from build123d import *

# Parameters (mm, degrees)
SKETCH_1_W                   = 80
SKETCH_1_H                   = 105
SKETCH_1_R                   = 4.5
EXTRUDE_1_DEPTH              = 15
HOLE_WIZARD_M8_1_D           = 6.8
HOLE_WIZARD_M8_1_DEPTH       = 22.25
HOLE_WIZARD_M8_1_CSINK_D     = 8.05
HOLE_WIZARD_M8_1_CSINK_ANGLE = 90
HOLE_WIZARD_M8_1_TIP         = 2.042926105


with BuildPart() as part:
    # 草图1 → 凸台-拉伸1 (new body)
    with BuildSketch(Plane.XY):
        Rectangle(SKETCH_1_W, SKETCH_1_H)
        with Locations((-30, -12.5)):
            Circle(SKETCH_1_R, mode=Mode.SUBTRACT)
        with Locations((30, -12.5)):
            Circle(SKETCH_1_R, mode=Mode.SUBTRACT)
        with Locations((30, -42.5)):
            Circle(SKETCH_1_R, mode=Mode.SUBTRACT)
        with Locations((-30, -42.5)):
            Circle(SKETCH_1_R, mode=Mode.SUBTRACT)
    extrude(amount=EXTRUDE_1_DEPTH)

    # M8 螺纹孔1
    with Locations(Plane(origin=(-32, 52.5, 7.5), x_dir=(0, 0, 1), z_dir=(0, 1, 0))):
        with Locations((0, 0), (0, 64)):
            CounterSinkHole(HOLE_WIZARD_M8_1_D / 2, HOLE_WIZARD_M8_1_CSINK_D / 2, depth=HOLE_WIZARD_M8_1_DEPTH, counter_sink_angle=HOLE_WIZARD_M8_1_CSINK_ANGLE)
            with Locations((0, 0, -(HOLE_WIZARD_M8_1_DEPTH + HOLE_WIZARD_M8_1_TIP / 2))):  # 118° drill point
                Cone(0, HOLE_WIZARD_M8_1_D / 2, HOLE_WIZARD_M8_1_TIP, mode=Mode.SUBTRACT)


solid = part.part
Read the model definition and answer for the solid it produces. Units are mm, in the model's axes. A direction names the side the tool comes from. Round coordinates to 2 decimals unless told otherwise and drop trailing zeros. Order: outer loops, then holes, each group sorted by start corner. A loop starts at its lowest first (then second) coordinate and runs counter-clockwise, first axis right, second up.
1) Flat-ended cylindrical pins translate along their axes: pin 1 (8 mm diameter, centred on x = -30, y = -42.5, fed in from -Z); pin 2 (8 mm diameter, centred on x = 32, z = 7.5, fed in from +Y) (3 decimals); pin 3 (14.5 mm diameter, centred on x = 30, y = -42.5, fed in from -Z); pin 4 (1 mm diameter, centred on x = 30.5, z = 8.5, fed in from +Y). Find the tip coordinate at first contact, or state that the pin passes through.
2) The part is cut by section D-D on x = -30. Give the number of separate pieces and of enclosed holes in the cut face, plus the area to 3 significant figures.
3) The mould has two halves that part along Y. Classify faces 1 (the face through (-1, 1, 0)), 2 (the face through (-1, 52.5, 7)), 3 (the face through (-27.92, -46.49, 7.4)): released by +Y, released by -Y, zero draft, split by the parting line, or undercut.
4) The part is cut by section A-A on y = 37.5. Write down the section's boundary in (x, z).
5) The part is cut by section C-C on y = -42.5. Write down the section's boundary in (x, z).
6) The part is cut by section B-B on z = 13. Write down the section's boundary in (x, y), plus the area to 3 significant figures.
7) For faces 4 (the face through (32.08, -46.49, 7.4)), 5 (the face through (29, 40.9, 5.9)), determine the directions among +Z, -Z, +X, -X, +Y, -Y from which every point of the face is accessible in a straight line to the end or side of a thin tool.
8) Straight lines are drawn through the part: L1, parallel to X at y = 46.75, z = 7.5; L2, parallel to X at y = -45.5, z = 6; L3, parallel to Y at x = -27, z = 5.75. For each, find the intervals that lie inside material, in ascending order.
Resolved:
1. pin 1: passes through
1. pin 2: stops at y = 52.475
1. pin 3: stops at z = 0
1. pin 4: stops at y = 29.59
2. separate pieces: 3
2. enclosed holes: 0
2. area: 1,180 mm2
3. face 1: zero draft
3. face 2: released by +Y
3. face 3: undercut
4. outline: (-40, 0) - (40, 0) - (40, 15) - (-40, 15) - close; hole circle Ø6.8 at (-32, 7.5); hole circle Ø6.8 at (32, 7.5)
5. outline: (-40, 0) - (-34.5, 0) - (-34.5, 15) - (-40, 15) - close; (-25.5, 0) - (25.5, 0) - (25.5, 15) - (-25.5, 15) - close; (34.5, 0) - (40, 0) - (40, 15) - (34.5, 15) - close
6. outline: (-40, -52.5) - (40, -52.5) - (40, 52.5) - (-40, 52.5) - close; hole circle Ø9 at (-30, -42.5); hole circle Ø9 at (-30, -12.5); hole circle Ø9 at (30, -42.5); hole circle Ø9 at (30, -12.5)
6. area: 8,150 mm2
7. face 4: +Z, -Z
7. face 5: +Y
8. L1: x = -40 to -35.4, -28.6 to 28.6, 35.4 to 40
8. L2: x = -40 to -33.35, -26.65 to 26.65, 33.35 to 40
8. L3: y = -52.5 to -45.85, -39.15 to -15.85, -9.15 to 52.5
